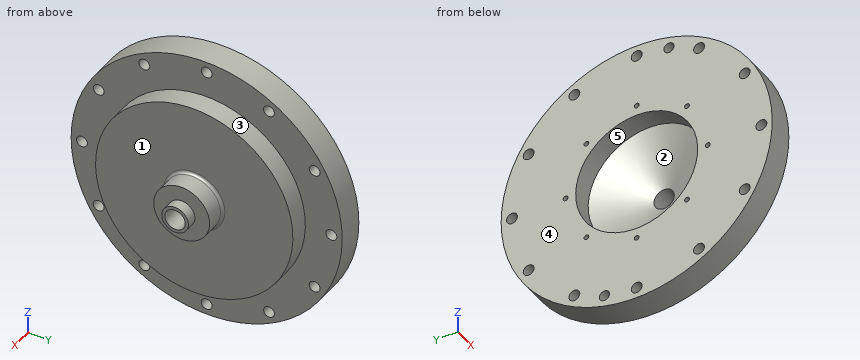
from build123d import *

# Parameters (mm, degrees)
SKETCH3_R                 = 4.7625
OXIDIZER_INLET_HOLE_DEPTH = 37.83
FLANGE_HOLES_D            = 5.1054
FLANGE_HOLES_DEPTH        = 22.225
DOWEL_HOLES_D             = 4.7625
DOWEL_HOLES_DEPTH         = 6.35
DOWEL_HOLES_TIP           = 1.430799349
SKETCH12_R                = 28.575
CUT_EXTRUDE2_DEPTH        = 9.525
SKETCH16_R                = 28.575
SKETCH17_R                = 4.7625
CIRPATTERN1_COUNT         = 8
FILLET1_R                 = 1.27
SKETCH25_OUTSIDE_W        = 165.668
SKETCH25_OUTSIDE_H        = 165.668
SKETCH25_OUTSIDE_R        = 46.228
CUT_EXTRUDE3_DEPTH        = 9.525


with BuildPart() as part:
    # Sketch2 → Main Structure (revolve)
    with BuildSketch(Plane.XY):
        Polygon((41.355, 13.081), (41.355, 6.2484), (46.355, 6.2484), (46.355, 0), (9.525, 0), (9.525, 63.5), (31.75, 63.5), (31.75, 13.081), align=None)
    revolve(axis=Axis((9.525, 0, 0), (1, 0, 0)))

    # Sketch3 → Oxidizer Inlet Hole (cut, through all)
    with BuildSketch(Plane(origin=(46.355, 0, 0), x_dir=(0, 0, -1), z_dir=(1, 0, 0))):
        Circle(SKETCH3_R)
    extrude(amount=-OXIDIZER_INLET_HOLE_DEPTH, mode=Mode.SUBTRACT)

    # Flange Holes
    with Locations(Plane(origin=(31.75, 0, 0), x_dir=(0, 0, 1), z_dir=(1, 0, 0))):
        with Locations((0, 58.42), (-29.21, 50.593204089), (-50.593204089, 29.21), (-58.42, 0), (-50.593204089, -29.21), (-29.21, -50.593204089), (0, -58.42), (29.21, -50.593204089), (50.593204089, -29.21), (58.42, 0), (50.593204089, 29.21), (29.21, 50.593204089)):
            Hole(FLANGE_HOLES_D / 2, depth=FLANGE_HOLES_DEPTH)

    # Dowel Holes
    with Locations(Plane.ZY.offset(-9.525)):
        with Locations((56.429386772, -15.120208615), (-56.429386772, 15.120208615)):
            Hole(DOWEL_HOLES_D / 2, depth=DOWEL_HOLES_DEPTH)
            with Locations((0, 0, -(DOWEL_HOLES_DEPTH + DOWEL_HOLES_TIP / 2))):  # 118° drill point
                Cone(0, DOWEL_HOLES_D / 2, DOWEL_HOLES_TIP, mode=Mode.SUBTRACT)

    # Sketch12 → Cut-Extrude2 (cut)
    with BuildSketch(Plane.ZY.offset(-9.525)):
        Circle(SKETCH12_R)
    extrude(amount=-CUT_EXTRUDE2_DEPTH, mode=Mode.SUBTRACT)

    # Sketch16 → Internal Flow Path Loft Cut section 0
    with BuildSketch(Plane.ZY.offset(-19.05)):
        Circle(SKETCH16_R)
    # Sketch17 → Internal Flow Path Loft Cut section 1
    with BuildSketch(Plane.ZY.offset(-30.48)):
        Circle(SKETCH17_R)
    loft(mode=Mode.SUBTRACT)

    # Sketch20 → #4-40 Tapped Hole1 (revolve, cut)
    with BuildSketch(Plane(origin=(9.525, 0, 33.3375), x_dir=(0, 0, 1), z_dir=(0, 1, 0))):
        Polygon((0, 0), (0, 13.887152758), (1.1303, 13.208), (1.1303, 0), align=None)
    f_4_40_tapped_hole1 = revolve(axis=Axis((3.175, 0, 33.3375), (1, 0, 0)), mode=Mode.SUBTRACT)

    # CirPattern1: #4-40 Tapped Hole1 ×8 about axis
    cirpattern1_axis = Axis((0, 0, 0), (1, 0, 0))
    for i in range(1, CIRPATTERN1_COUNT):
        add(f_4_40_tapped_hole1.rotate(cirpattern1_axis, i * 360 / CIRPATTERN1_COUNT), mode=Mode.SUBTRACT)

    # Fillet1
    fillet1_edges = [part.edges().sort_by_distance(p)[0] for p in [
        (31.75, -13.081, 0),
    ]]
    fillet(fillet1_edges, radius=FILLET1_R)

    # Sketch25 outside → Cut-Extrude3 (cut)
    with BuildSketch(Plane(origin=(31.75, 0, 0), x_dir=(0, 0, -1), z_dir=(1, 0, 0))):
        Rectangle(SKETCH25_OUTSIDE_W, SKETCH25_OUTSIDE_H)
        Circle(SKETCH25_OUTSIDE_R, mode=Mode.SUBTRACT)
    extrude(amount=-CUT_EXTRUDE3_DEPTH, mode=Mode.SUBTRACT)


solid = part.part
Geometry: final body of the model. Coordinates: model frame, mm. Face numbers are marked on the shaded views. A direction names the side the tool comes from. Give positions to 0.01 mm unless a question says otherwise; leave off trailing zeros. Loops run counter-clockwise (first coordinate to the right, second up) from the corner with the lowest first, then second, coordinate; pieces in that order, holes last. Notation, with made-up numbers: (25, 8.25) - (71, 8.25) arc R20 ccw to (71, 37.25) - close; hole circle Ø8 at (-36.75, 35). An arc over 180 degrees is marked (long way). One line per question, with ' | ' between items. Start each with the question number.
(1) Contact query for flat-ended pins moving along their axis: pin 1 (2 mm diameter, centred on y = 33.34, z = 0, fed in from +X); pin 2 (2 mm diameter, centred on y = -33.34, z = 0, fed in from -X); pin 3 (5 mm diameter, centred on x = 42, z = -3.5, fed in from -Y). Output: stop coordinate, or through.
(2) Reachability of the marked faces 1 and 2 from +Z, -Z, +X, -X, +Y, -Y: full face, straight path, thin tool, end or side. Return the list, or none.
(3) Section query A-A on y = 58.42. Return loops of the section in (x, z) (3 decimals), then the cut area to 3 significant figures.
(4) Ray query, line 1 (Y direction, x = 22, z = -23.5); line 2 (Z direction, x = 14, y = -29). Return the intervals inside material, ascending. Write a range as from..to.
(5) Section query C-C on x = 43. Return loops of the section in (y, z) (1 decimal), then the cut area to 3 significant figures.
(6) Pull-direction query (Z, two-part tool) for the marked faces 3, 4 and 5; classes: released by +Z, released by -Z, zero draft, split by the parting line, or undercut.
(7) Section query B-B on z = 41. Return loops of the section in (x, y) (3 decimals), then the cut area to 3 significant figures.
The answers:
1) pin 1: x = 31.75 | pin 2: x = 22.81 | pin 3: y = -13.04
2) face 1: +X | face 2: -X
3) outline: (9.525, -24.887) - (22.225, -24.887) - (22.225, -2.553) - (9.525, -2.553) - close; (9.525, 2.553) - (22.225, 2.553) - (22.225, 24.887) - (9.525, 24.887) - close | area: 567 mm2
4) line 1: -58.99..-24.7, -22.45..22.45, 24.7..58.99 | line 2: -56.49..-53.14, -48.05..48.05, 53.14..56.49
5) outline: circle Ø12.5 at (0, 0); hole circle Ø9.5 at (0, 0) | area: 51.4 mm2
6) face 3: split by the parting line | face 4: zero draft | face 5: undercut
7) outline: (9.525, -48.49) - (22.225, -48.49) - (22.225, -21.355) - (31.75, -21.355) - (31.75, 21.355) - (22.225, 21.355) - (22.225, 48.49) - (9.525, 48.49) - close | area: 1,640 mm2
